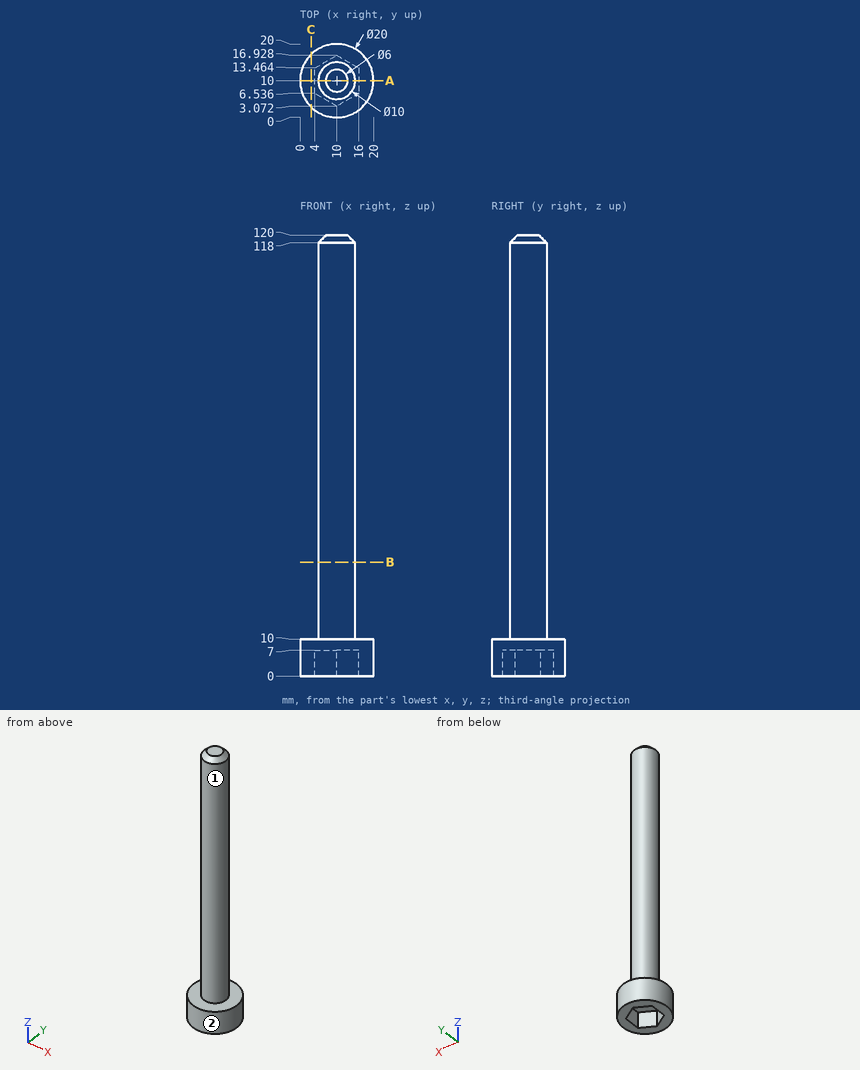
Job drawing, mm, ordinate dimensions from the low corner. One solid piece. A direction names the side the tool comes from. Coordinates: 2 decimals unless noted, no trailing zeros. Write each loop counter-clockwise with the first axis right and the second up, starting at its lowest first coordinate (ties: lowest second). Pieces come first, ordered by that corner, then holes. Notation, with made-up numbers: M 29.25,-7 L 69.25,-7 A7 cw 69.25,2 Z; hole C -11,19.5 d1. An arc over 180 degrees is marked long. Answer as a JSON object with one key per item and string values. Group by question number.
1) Wall check: line 1 (Z direction, x = 12.75, y = 5.75); line 2 (X direction, y = 10.25, z = 17); line 3 (Z direction, x = 10.5, y = 9). Give the ranges that are in metal, low to high. Write a range as from..to.
2) Pin check, flat tips, straight feed: pin 1 Ø10 at (y, z) = (10, 98.5) entering from +X; pin 2 Ø10 at (y, z) = (16, 69.5) entering from -X; pin 3 Ø2 at (y, z) = (11.5, 2) entering from -X. Stop position of each tip, or through.
3) Tool access for the marked faces 1 and 2: list every direction of +Z, -Z, +X, -X, +Y, -Y with a clear straight run to the whole face (end or side of a thin tool).
4) Saw through at B-B (z = 31). Write the cut outline in (x, y).
5) Saw through at A-A (y = 10). Write the cut outline in (x, z).
6) Saw through at C-C (x = 3). Write the cut outline in (y, z).
Values follow:
{
 "1": {"line 1": "z = 7..10", "line 2": "x = 5.01..14.99", "line 3": "z = 7..120"},
 "2": {"pin 1": "stops at x = 15", "pin 2": "stops at x = 5.1", "pin 3": "stops at x = 0.01"},
 "3": {"face 1": "+Z", "face 2": "+Z, -Z"},
 "4": {"outline": "C 10,10 d10"},
 "5": {"outline": "M 0,0 L 4,0 L 4,7 L 16,7 L 16,0 L 20,0 L 20,10 L 15,10 L 15,118 L 13,120 L 7,120 L 5,118 L 5,10 L 0,10 Z"},
 "6": {"outline": "M 2.86,0 L 17.14,0 L 17.14,10 L 2.86,10 Z"}
}
